```python
from build123d import *

# Parameters (mm, degrees)
SKETCH1_R           = 30
SKETCH1_R_2         = 7
BOSS_EXTRUDE1_DEPTH = 10
FILLET1_R           = 10
FILLET2_R           = 20
CUT_EXTRUDE4_DEPTH  = 21
BOSS_EXTRUDE2_DEPTH = 2.5
CUT_EXTRUDE3_DEPTH  = 21


with BuildPart() as part:
    # Sketch1 → Boss-Extrude1 (new body, symmetric)
    with BuildSketch(Plane(origin=(0, 0, 0), x_dir=(1, 0, 0), z_dir=(0, 1, 0))):
        with BuildLine():
            Line((27.935473676, 25.760615491), (128.063755469, 9.084385863))
            ThreePointArc((128.063755469, 9.084385863), (155, 0), (128.063755469, -9.084385863))
            Line((128.063755469, -9.084385863), (27.935473676, -25.760615491))
            ThreePointArc((27.935473676, -25.760615491), (-38, 0), (27.935473676, 25.760615491))
        make_face()
        Circle(SKETCH1_R, mode=Mode.SUBTRACT)
        with Locations((140, 0)):
            Circle(SKETCH1_R_2, mode=Mode.SUBTRACT)
    extrude(amount=BOSS_EXTRUDE1_DEPTH, both=True)

    # Fillet1
    fillet1_edges = [part.edges().sort_by_distance(p)[0] for p in [
        (128.063755469, 0, -9.084385863),
        (128.063755469, 0, 9.084385863),
    ]]
    fillet(fillet1_edges, radius=FILLET1_R)

    # Fillet2
    fillet2_edges = [part.edges().sort_by_distance(p)[0] for p in [
        (27.935473676, 0, -25.760615491),
        (27.935473676, 0, 25.760615491),
    ]]
    fillet(fillet2_edges, radius=FILLET2_R)

    # Sketch14 → Cut-Extrude4 (cut, through all)
    with BuildSketch(Plane(origin=(0, 10, 0), x_dir=(1, 0, 0), z_dir=(0, 1, 0))):
        with BuildLine():
            Line((41.828554558, 17.870982725), (122.478416149, 4.438857582))
            ThreePointArc((122.478416149, 4.438857582), (126.239130435, 0), (122.478416149, -4.438857582))
            Line((122.478416149, -4.438857582), (41.828554558, -17.870982725))
            ThreePointArc((41.828554558, -17.870982725), (37.231968897, -16.217361812), (36.238855523, -11.43439331))
            ThreePointArc((36.238855523, -11.43439331), (38, 0), (36.238855523, 11.43439331))
            ThreePointArc((36.238855523, 11.43439331), (37.231968897, 16.217361812), (41.828554558, 17.870982725))
        make_face()
    extrude(amount=-CUT_EXTRUDE4_DEPTH, mode=Mode.SUBTRACT)

    # Sketch11 → Boss-Extrude2 (add, symmetric)
    with BuildSketch(Plane(origin=(0, 0, 0), x_dir=(1, 0, 0), z_dir=(0, 1, 0))):
        with BuildLine():
            Line((41.828554558, 17.870982725), (122.478416149, 4.438857582))
            ThreePointArc((122.478416149, 4.438857582), (126.239130435, 0), (122.478416149, -4.438857582))
            Line((122.478416149, -4.438857582), (41.828554558, -17.870982725))
            ThreePointArc((41.828554558, -17.870982725), (37.231968897, -16.217361812), (36.238855523, -11.43439331))
            ThreePointArc((36.238855523, -11.43439331), (38, 0), (36.238855523, 11.43439331))
            ThreePointArc((36.238855523, 11.43439331), (37.231968897, 16.217361812), (41.828554558, 17.870982725))
        make_face()
    extrude(amount=BOSS_EXTRUDE2_DEPTH, both=True)

    # Sketch2 → Cut-Extrude3 (cut, through all)
    with BuildSketch(Plane(origin=(0, 10, 0), x_dir=(1, 0, 0), z_dir=(0, 1, 0))):
        with BuildLine():
            Line((74.800916149, 12.37948059), (82.190906374, 11.148687733))
            ThreePointArc((82.190906374, 11.148687733), (91.636361303, 0), (82.190906374, -11.148687733))
            Line((82.190906374, -11.148687733), (74.800916149, -12.37948059))
            ThreePointArc((74.800916149, -12.37948059), (60.189130435, 0), (74.800916149, 12.37948059))
        make_face()
    extrude(amount=-CUT_EXTRUDE3_DEPTH, mode=Mode.SUBTRACT)


solid = part.part
```
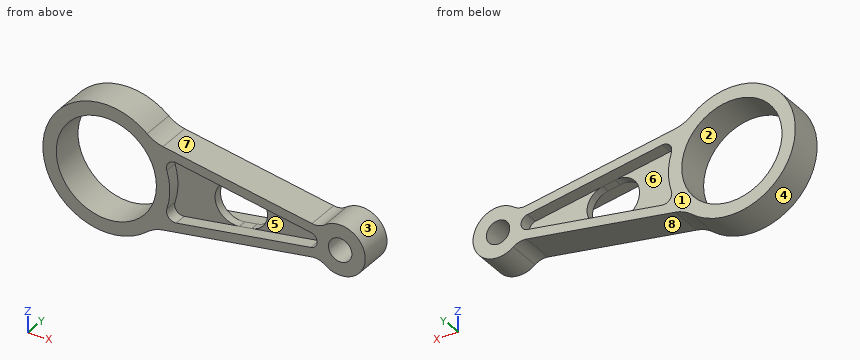
Model file for the job. Use its own axes, mm. Face numbers are marked on the shaded views. A direction names the side the tool comes from. Coordinates: 2 decimals unless noted, no trailing zeros. Order: outer loops, then holes, each group sorted by start corner. A loop starts at its lowest first (then second) coordinate and runs counter-clockwise, first axis right, second up. Notation, with made-up numbers: (45, -24) -> (56, -24) arc R10 ccw to (56, -20) -> close; hole circle Ø9 at (83.25, 71). An arc over 180 degrees is marked (long way). Answer as a JSON object with one key per item and string values. Group by question number.
1) Which spindle directions (+Z, -Z, +X, -X, +Y, -Y) get a long thin tool onto all of the face, cutting with end or side? Do the marked faces 4, 5, 6, 7 and 8. Say none if no direction does.
2) Cut at B-B, the plane y = -6.5. Write the cut outline in (x, z), then the cut area to 3 significant figures.
3) Cut at C-C, the plane x = 140. Write the cut outline in (y, z).
4) Cut at A-A, the plane z = 0. Write the cut outline in (x, y).
5) Flat gauge pins, fed straight in: pin 1 (1 mm diameter, centred on x = 73, y = -3, fed in from +Z); pin 2 (10 mm diameter, centred on x = 46, y = -8, fed in from -Z); pin 3 (1.5 mm diameter, centred on y = 0, z = -11.5, fed in from -X); pin 4 (18 mm diameter, centred on x = 99.5, z = 5.5, fed in from -Y). Where does each tip first touch, or does it go through?
6) Cut at D-D, the plane x = 46. Write the cut outline in (y, z), then the cut area to 3 significant figures.
7) Pull direction Z, two halves, no side cores. Call the marked faces 1, 2 and 3: +Z half, -Z half, draft (parallel to the pull), parting line (faces both ways), or undercut.
8) Drill centre lines: L1, parallel to X at y = 7, z = -0.5; L2, parallel to Z at x = 140, y = -1; L3, parallel to Z at x = 0, y = 0.75. Where is each one in solid material? Low to high.
Check values:
{
 "1": {"face 4": "+Y, -Y", "face 5": "-Y", "face 6": "+Y", "face 7": "+Z, +Y, -Y", "face 8": "-Z, +Y, -Y"},
 "2": {"outline": "(24.38, -29.15) arc R20 cw to (33.92, -24.76) -> (123.07, -9.92) arc R10 cw to (130.83, -11.87) arc R15 ccw (long way) to (130.83, 11.87) arc R10 cw to (123.07, 9.92) -> (33.92, 24.76) arc R20 cw to (24.38, 29.15) arc R38 ccw (long way) to start; hole circle Ø60 at (0, 0); hole (36.24, -11.43) arc R5 ccw to (41.83, -17.87) -> (122.48, -4.44) arc R4.5 ccw to (122.48, 4.44) -> (41.83, 17.87) arc R5 ccw to (36.24, 11.43) arc R38 cw to start; hole circle Ø14 at (140, 0)", "area": "3,380 mm²"},
 "3": {"outline": "(-10, -15) -> (10, -15) -> (10, -7) -> (-10, -7) -> close; (-10, 7) -> (10, 7) -> (10, 15) -> (-10, 15) -> close"},
 "4": {"outline": "(-38, -10) -> (-30, -10) -> (-30, 10) -> (-38, 10) -> close; (30, -10) -> (38, -10) -> (38, -2.5) -> (60.19, -2.5) -> (60.19, 2.5) -> (38, 2.5) -> (38, 10) -> (30, 10) -> close; (91.64, -2.5) -> (126.24, -2.5) -> (126.24, -10) -> (133, -10) -> (133, 10) -> (126.24, 10) -> (126.24, 2.5) -> (91.64, 2.5) -> close; (147, -10) -> (155, -10) -> (155, 10) -> (147, 10) -> close"},
 "5": {"pin 1": "stops at z = 18.34", "pin 2": "stops at z = -23.58", "pin 3": "stops at x = -36.45", "pin 4": "stops at y = -10"},
 "6": {"outline": "(-10, -22.75) -> (10, -22.75) -> (10, -17.18) -> (2.5, -17.18) -> (2.5, 17.18) -> (10, 17.18) -> (10, 22.75) -> (-10, 22.75) -> (-10, 17.18) -> (-2.5, 17.18) -> (-2.5, -17.18) -> (-10, -17.18) -> close", "area": "395 mm²"},
 "7": {"face 1": "draft", "face 2": "undercut", "face 3": "parting line"},
 "8": {"L1": "x = -38 to -30, 30 to 38, 126.21 to 133.02, 146.98 to 154.99", "L2": "z = -15 to -7, 7 to 15", "L3": "z = -38 to -30, 30 to 38"}
}
